from build123d import *

# Parameters (mm, degrees)
SKETCH1_W           = 89
SKETCH1_H           = 89
BOSS_EXTRUDE1_DEPTH = 2
SKETCH2_W           = 10
SKETCH2_H           = 10
BOSS_EXTRUDE2_DEPTH = 2
SKETCH3_W           = 10
SKETCH3_H           = 3
SKETCH3_W_2         = 3
SKETCH3_H_2         = 10
BOSS_EXTRUDE3_DEPTH = 0.2
FILLET1_R           = 2


with BuildPart() as part:
    # Sketch1 → Boss-Extrude1 (new body)
    with BuildSketch(Plane(origin=(0, 0, 0), x_dir=(1, 0, 0), z_dir=(0, 1, 0))):
        Rectangle(SKETCH1_W, SKETCH1_H)
    extrude(amount=BOSS_EXTRUDE1_DEPTH)

    # Sketch2 → Boss-Extrude2 (add)
    with BuildSketch(Plane(origin=(0, 2, 0), x_dir=(1, 0, 0), z_dir=(0, 1, 0))):
        with Locations((-39.5, 39.5)):
            Rectangle(SKETCH2_W, SKETCH2_H)
        with Locations((39.5, 39.5)):
            Rectangle(SKETCH2_W, SKETCH2_H)
        with Locations((39.5, -39.5)):
            Rectangle(SKETCH2_W, SKETCH2_H)
        with Locations((-39.5, -39.5)):
            Rectangle(SKETCH2_W, SKETCH2_H)
    extrude(amount=BOSS_EXTRUDE2_DEPTH)

    # Sketch3 → Boss-Extrude3 (add)
    with BuildSketch(Plane(origin=(0, 2, 0), x_dir=(1, 0, 0), z_dir=(0, 1, 0))):
        with Locations((-39.5, 30)):
            Rectangle(SKETCH3_W, SKETCH3_H)
        with Locations((-30, 39.5)):
            Rectangle(SKETCH3_W_2, SKETCH3_H_2)
        with Locations((-39.5, 24)):
            Rectangle(SKETCH3_W, SKETCH3_H)
        with Locations((-24, 39.5)):
            Rectangle(SKETCH3_W_2, SKETCH3_H_2)
        with Locations((-39.5, 18)):
            Rectangle(SKETCH3_W, SKETCH3_H)
        with Locations((-18, 39.5)):
            Rectangle(SKETCH3_W_2, SKETCH3_H_2)
        with Locations((-39.5, 12)):
            Rectangle(SKETCH3_W, SKETCH3_H)
        with Locations((-12, 39.5)):
            Rectangle(SKETCH3_W_2, SKETCH3_H_2)
        with Locations((-39.5, 6)):
            Rectangle(SKETCH3_W, SKETCH3_H)
        with Locations((-6, 39.5)):
            Rectangle(SKETCH3_W_2, SKETCH3_H_2)
        with Locations((-39.5, 0)):
            Rectangle(SKETCH3_W, SKETCH3_H)
        with Locations((0, 39.5)):
            Rectangle(SKETCH3_W_2, SKETCH3_H_2)
        with Locations((-39.5, -6)):
            Rectangle(SKETCH3_W, SKETCH3_H)
        with Locations((6, 39.5)):
            Rectangle(SKETCH3_W_2, SKETCH3_H_2)
        with Locations((-39.5, -12)):
            Rectangle(SKETCH3_W, SKETCH3_H)
        with Locations((12, 39.5)):
            Rectangle(SKETCH3_W_2, SKETCH3_H_2)
        with Locations((-39.5, -18)):
            Rectangle(SKETCH3_W, SKETCH3_H)
        with Locations((18, 39.5)):
            Rectangle(SKETCH3_W_2, SKETCH3_H_2)
        with Locations((-39.5, -24)):
            Rectangle(SKETCH3_W, SKETCH3_H)
        with Locations((24, 39.5)):
            Rectangle(SKETCH3_W_2, SKETCH3_H_2)
        with Locations((-39.5, -30)):
            Rectangle(SKETCH3_W, SKETCH3_H)
        with Locations((30, 39.5)):
            Rectangle(SKETCH3_W_2, SKETCH3_H_2)
        with Locations((-30, -39.5)):
            Rectangle(SKETCH3_W_2, SKETCH3_H_2)
        with Locations((39.5, 30)):
            Rectangle(SKETCH3_W, SKETCH3_H)
        with Locations((-24, -39.5)):
            Rectangle(SKETCH3_W_2, SKETCH3_H_2)
        with Locations((39.5, 24)):
            Rectangle(SKETCH3_W, SKETCH3_H)
        with Locations((-18, -39.5)):
            Rectangle(SKETCH3_W_2, SKETCH3_H_2)
        with Locations((39.5, 18)):
            Rectangle(SKETCH3_W, SKETCH3_H)
        with Locations((-12, -39.5)):
            Rectangle(SKETCH3_W_2, SKETCH3_H_2)
        with Locations((39.5, 12)):
            Rectangle(SKETCH3_W, SKETCH3_H)
        with Locations((-6, -39.5)):
            Rectangle(SKETCH3_W_2, SKETCH3_H_2)
        with Locations((39.5, 6)):
            Rectangle(SKETCH3_W, SKETCH3_H)
        with Locations((0, -39.5)):
            Rectangle(SKETCH3_W_2, SKETCH3_H_2)
        with Locations((39.5, 0)):
            Rectangle(SKETCH3_W, SKETCH3_H)
        with Locations((6, -39.5)):
            Rectangle(SKETCH3_W_2, SKETCH3_H_2)
        with Locations((39.5, -6)):
            Rectangle(SKETCH3_W, SKETCH3_H)
        with Locations((12, -39.5)):
            Rectangle(SKETCH3_W_2, SKETCH3_H_2)
        with Locations((39.5, -12)):
            Rectangle(SKETCH3_W, SKETCH3_H)
        with Locations((18, -39.5)):
            Rectangle(SKETCH3_W_2, SKETCH3_H_2)
        with Locations((39.5, -18)):
            Rectangle(SKETCH3_W, SKETCH3_H)
        with Locations((24, -39.5)):
            Rectangle(SKETCH3_W_2, SKETCH3_H_2)
        with Locations((39.5, -24)):
            Rectangle(SKETCH3_W, SKETCH3_H)
        with Locations((30, -39.5)):
            Rectangle(SKETCH3_W_2, SKETCH3_H_2)
        with Locations((39.5, -30)):
            Rectangle(SKETCH3_W, SKETCH3_H)
    extrude(amount=BOSS_EXTRUDE3_DEPTH)

    # Fillet1
    fillet1_edges = [part.edges().sort_by_distance(p)[0] for p in [
        (-34.5, 3, -34.5),
        (34.5, 3, -34.5),
        (34.5, 3, 34.5),
        (-34.5, 3, 34.5),
    ]]
    fillet(fillet1_edges, radius=FILLET1_R)


solid = part.part
Source: CAD feature listing. Evaluate the final solid. Frame: model axes, mm. A direction names the side the tool comes from. Give positions to 0.01 mm unless a question says otherwise; leave off trailing zeros. Write each loop counter-clockwise with the first axis right and the second up, starting at its lowest first coordinate (ties: lowest second). Pieces come first, ordered by that corner, then holes. Notation, with made-up numbers: (24, -0.75) -> (59, -0.75) arc R31 ccw to (59, 38.25) -> close; hole circle Ø2 at (51.25, -22). An arc over 180 degrees is marked (long way). Write item = value, one per line.
Q1. Reachability of faces 4 (the face through (-34.5, 3, 41)), 5 (the face through (39, 2.2, -18)), 6 (the face through (-40, 4, -40)) from +Z, -Z, +X, -X, +Y, -Y: full face, straight path, thin tool, end or side. Return the list, or none.
Here are the results:
face_4 = +Z, -Z, +Y
face_5 = +X, -X, +Y
face_6 = +Z, -Z, +X, -X, +Y
Q2. Mould query, pull axis X, two halves, no side actions, for faces 1 (the face through (-35.1, 3.01, 35.07)), 2 (the face through (39, 2.2, -30)), 3 (the face through (44.5, 2, 1)). Classes: +X half, -X half, draft (parallel to the pull), parting line (faces both ways), or undercut.
Here are the results:
face_1 = undercut
face_2 = draft
face_3 = +X half
Q3. Cut plane B-B on x = -24. Return loops of the section in (y, z), then the cut area to 3 significant figures.
Here are the results:
outline = (0, -44.5) -> (2.2, -44.5) -> (2.2, -34.5) -> (2, -34.5) -> (2, 34.5) -> (2.2, 34.5) -> (2.2, 44.5) -> (0, 44.5) -> close
area = 182 mm²
Q4. Line query: line 1 (X direction, y = 3.05, z = 37); line 2 (Y direction, x = -1.5, z = 15.5). Output: solid intervals per line, ascending. Write a range as from..to.
Here are the results:
line_1 = -44.5..-34.5, 34.5..44.5
line_2 = 0..2
Q5. First-contact query: pin 1 (2.5 mm diameter, centred on x = -39, z = 11.5, fed in from +Y); pin 2 (6 mm diameter, centred on x = 20, z = -17, fed in from +Y). Flat tips, straight axial feed; report the tip coordinate or a pass-through.
Here are the results:
pin_1 = 2.2
pin_2 = 2
Q6. Cut plane A-A on y = 3.3. Return loops of the section in (x, z).
Here are the results:
outline = (-44.5, -44.5) -> (-34.5, -44.5) -> (-34.5, -36.5) arc R2 ccw to (-36.5, -34.5) -> (-44.5, -34.5) -> close; (-44.5, 34.5) -> (-36.5, 34.5) arc R2 ccw to (-34.5, 36.5) -> (-34.5, 44.5) -> (-44.5, 44.5) -> close; (34.5, -44.5) -> (44.5, -44.5) -> (44.5, -34.5) -> (36.5, -34.5) arc R2 ccw to (34.5, -36.5) -> close; (34.5, 36.5) arc R2 ccw to (36.5, 34.5) -> (44.5, 34.5) -> (44.5, 44.5) -> (34.5, 44.5) -> close
